```python
from build123d import *

# Parameters (mm, degrees)
BOSS_EXTRUDE1_DEPTH = 48
CUT_EXTRUDE1_DEPTH  = 34
SKETCH4_W           = 34
SKETCH4_H           = 5.062205584
BOSS_EXTRUDE2_DEPTH = 10
SKETCH6_W           = 34
SKETCH6_H           = 31
CUT_EXTRUDE3_DEPTH  = 101.30083919
BOSS_EXTRUDE3_DEPTH = 34
SKETCH9_W           = 34
SKETCH9_H           = 5.06
BOSS_EXTRUDE4_DEPTH = 10
BOSS_EXTRUDE5_DEPTH = 5


with BuildPart() as part:
    # Sketch1 → Boss-Extrude1 (new body)
    with BuildSketch(Plane(origin=(0, 0, 0), x_dir=(0, 0, -1), z_dir=(1, 0, 0))):
        with BuildLine():
            Line((-22.763988027, 0), (-22.763988027, 8.659101585))
            Line((-22.763988027, 8.659101585), (-8.763988027, 40))
            Line((-8.763988027, 40), (-8.763988027, 58))
            Line((-8.763988027, 58), (51.236011973, 58))
            Line((51.236011973, 58), (51.236011973, 40))
            Line((51.236011973, 40), (65.236011973, 8.659101585))
            Line((65.236011973, 8.659101585), (65.236011973, 0))
            Line((65.236011973, 0), (45.236011973, 0))
            Line((45.236011973, 0), (45.236011973, 12))
            Line((45.236011973, 12), (41.236011973, 12))
            ThreePointArc((41.236011973, 12), (21.236011973, 32), (1.236011973, 12))
            Line((1.236011973, 12), (-2.763988027, 12))
            Line((-2.763988027, 12), (-2.763988027, 0))
            Line((-2.763988027, 0), (-22.763988027, 0))
        make_face()
    extrude(amount=-BOSS_EXTRUDE1_DEPTH)

    # Sketch3 → Cut-Extrude1 (cut)
    with BuildSketch(Plane(origin=(-7, 0, 0), x_dir=(0, 0, -1), z_dir=(1, 0, 0))):
        Polygon((-19.038103202, 17), (-1.038103202, 17), (-1.038103202, 58), (-8.763988027, 58), (-8.763988027, 40), align=None)
    extrude(amount=-CUT_EXTRUDE1_DEPTH, mode=Mode.SUBTRACT)

    # Sketch4 → Boss-Extrude2 (add)
    with BuildSketch(Plane(origin=(0, 17, 0), x_dir=(1, 0, 0), z_dir=(0, 1, 0))):
        with Locations((-24, -3.569205994)):
            Rectangle(SKETCH4_W, SKETCH4_H)
    extrude(amount=BOSS_EXTRUDE2_DEPTH)

    # Sketch6 → Cut-Extrude3 (cut, through all)
    with BuildSketch(Plane.XY.offset(1.038103202)):
        with Locations((-24, 42.5)):
            Rectangle(SKETCH6_W, SKETCH6_H)
    extrude(amount=-CUT_EXTRUDE3_DEPTH, mode=Mode.SUBTRACT)

    # Sketch8 → Boss-Extrude3 (add)
    with BuildSketch(Plane(origin=(-41, 0, 0), x_dir=(0, 0, -1), z_dir=(1, 0, 0))):
        with BuildLine():
            Line((-2.24605546, 27), (45.75394454, 27))
            ThreePointArc((45.75394454, 27), (21.75394454, 51), (-2.24605546, 27))
        make_face()
    extrude(amount=BOSS_EXTRUDE3_DEPTH)

    # Sketch9 → Boss-Extrude4 (add)
    with BuildSketch(Plane(origin=(0, 27, 0), x_dir=(1, 0, 0), z_dir=(0, 1, 0))):
        with Locations((-24, 46.107548199)):
            Rectangle(SKETCH9_W, SKETCH9_H)
    extrude(amount=BOSS_EXTRUDE4_DEPTH)

    # Sketch10 → Boss-Extrude5 (add)
    with BuildSketch(Plane(origin=(0, 58, 0), x_dir=(1, 0, 0), z_dir=(0, 1, 0))):
        Polygon((-41, 48.707326909), (-7, 48.637548199), (-7, -6.100308786), (-41, -6.100308786), align=None)
    extrude(amount=-BOSS_EXTRUDE5_DEPTH)


solid = part.part
```
Can you work these out from the model? Positions are in its coordinate system, mm. A direction names the side the tool comes from. Round coordinates to 2 decimals unless told otherwise and drop trailing zeros. Loops run counter-clockwise (first coordinate to the right, second up) from the corner with the lowest first, then second, coordinate; pieces in that order, holes last. Notation, with made-up numbers: M -21,-28 L 14,-28 A24 cw 14,-11 Z; hole C 62.25,26.25 d1. An arc over 180 degrees is marked long. Write item = value, one per line. Start each with the question number.
(1) Which directions (+Z, -Z, +X, -X, +Y, -Y) give clear straight access to the entire face, cutting with the end or side of a thin tool? Please do faces 5 (the face through (-24, 12, 1)), 6 (the face through (-41, 50, -10)), 7 (the face through (-3, 49, 8.764)), 8 (the face through (-3, 49, -51.236)).
(2) I'm going to push flat-ended pins straight in: P1, Ø3, axis at x = -28, z = 1.5, coming from the -Y side; P2, Ø6, axis at x = -8.5, y = 37.5, coming from the +Z side; P3, Ø3, axis at x = -7, y = 42, coming from the -Z side; P4, Ø12, axis at x = -42, y = 45.5, coming from the -Z side. Where does each tip first touch, or does it pass through?
(3) If we mould it in two halves opening along X, with no side actions, what happens to faces 1 (the face through (-24, 22, 6.1)), 2 (the face through (-24.238, 50.542, -17.09)), 3 (the face through (0, 36, -22)), 4 (the face through (-24, 58, -21))? For each: released by +X, released by -X, zero draft, split by the parting line, or undercut.
(4) I need wall thicknesses on line 1 along Z through (x, y) = (-42.5, 2.5); line 2 along X through (y, z) = (18, 16.5); line 3 along Z through (x, y) = (-6, 41). Which ranges of each line are inside material? Lowest first, please.
(5) Suppose I cut it at D-D on x = -4. Write out the boundary of the cut face in (y, z), plus the area to 3 significant figures.
(6) Suppose I cut it at A-A on z = 4. Write out the boundary of the cut face in (x, y), plus the area to 3 significant figures.
(7) Suppose I cut it at C-C on y = 16. Write out the boundary of the cut face in (x, z).
Answer block:
q1.face_5 = +X, -X, -Y
q1.face_6 = none
q1.face_7 = +Z, +X, -X, +Y
q1.face_8 = -Z, +X, -X, +Y
q2.P1 = 0
q2.P2 = 11.04
q2.P3 = -51.24
q2.P4 = -51.46
q3.face_1 = undercut
q3.face_2 = undercut
q3.face_3 = released by +X
q3.face_4 = zero draft
q4.line_1 = -65.24 to -45.24, 2.76 to 22.76
q4.line_2 = -48 to -41, -7 to 0
q4.line_3 = -51.24 to 8.76
q5.outline = M 0,-65.24 L 8.66,-65.24 L 40,-51.24 L 58,-51.24 L 58,8.76 L 40,8.76 L 8.66,22.76 L 0,22.76 L 0,2.76 L 12,2.76 L 12,-1.24 A20 cw 12,-41.24 L 12,-45.24 L 0,-45.24 Z
q5.area = 2,960 mm²
q6.outline = M -48,0 L 0,0 L 0,58 L -48,58 Z; hole M -41,27 L -7,27 L -7,53 L -41,53 Z
q6.area = 1,900 mm²
q7.outline = M -48,-61.96 L 0,-61.96 L 0,-40.83 L -48,-40.83 Z; M -48,-1.64 L 0,-1.64 L 0,19.48 L -48,19.48 Z
